from build123d import *

# Parameters (mm, degrees)
BOSS_EXTRUDE1_DEPTH     = 6.35
CUT_EXTRUDE1_DEPTH      = 72.114330131
CUT_EXTRUDE1_DEPTH_BACK = 72.114330131
SKETCH2_R               = 3.175
SCALE1_SCALE            = 4


with BuildPart() as part:
    # Sketch1 → Boss-Extrude1 (new body)
    with BuildSketch(Plane.XY):
        with BuildLine():
            Line((-63.5, 6.985), (63.5, 6.985))
            ThreePointArc((63.5, 6.985), (70.485, 0), (63.5, -6.985))
            Line((63.5, -6.985), (-63.5, -6.985))
            ThreePointArc((-63.5, -6.985), (-70.485, 0), (-63.5, 6.985))
        make_face()
    extrude(amount=BOSS_EXTRUDE1_DEPTH)

    # Sketch2 → Cut-Extrude1 (cut, two sides: drawn at the far end of the back side and taken through both)
    with BuildSketch(Plane.XY.offset(6.35).offset(-CUT_EXTRUDE1_DEPTH_BACK)):
        with Locations((63.5, 0)):
            Circle(SKETCH2_R)
        with Locations((-63.5, 0)):
            Circle(SKETCH2_R)
    extrude(amount=CUT_EXTRUDE1_DEPTH + CUT_EXTRUDE1_DEPTH_BACK, mode=Mode.SUBTRACT)


with BuildPart() as part_1:
    # Scale1: scaled about (0, 0, 3.175)
    add(part.part.scale(SCALE1_SCALE).moved(Location((0, 0, -9.525))))


solid = part_1.part
Check sheet for the modelled part. Datum: model origin and axes. Units: mm. Round coordinates to 2 decimals unless told otherwise and drop trailing zeros. Order: outer loops, then holes, each group sorted by start corner. A loop starts at its lowest first (then second) coordinate and runs counter-clockwise, first axis right, second up. Notation, with made-up numbers: M 76.25,15 L 85.25,15 A19 cw 85.25,23 Z; hole C 77,-26.75 d6. An arc over 180 degrees is marked long. One line per item, written item: value. Start each with the question number.
1. Section check C-C on y = 21. Enter the section's corners in (x, z) (3 decimals).
2. Section check A-A on y = 0. Enter the section's corners in (x, z) (3 decimals).
3. Scan lines: line 1 along X through (y, z) = (-1, 14.25); line 2 along X through (y, z) = (-7.5, -0.25); line 3 along Y through (x, z) = (254, 4.75). Record each from-to range of solid material in increasing order.
4. Gauge pin test, flat ends, axial feed: P1, Ø8, axis at y = -19, z = 4.5, coming from the +X side; P2, Ø1, axis at y = 10, z = -3.5, coming from the -X side; P3, Ø1, axis at y = 7.5, z = 7.5, coming from the -X side. Record the tip position at first contact, or that the pin passes through.
5. Section check B-B on z = -4.5. Enter the section's corners in (x, y), and give its area (3 significant figures).
6. Release check for a two-part mould opening along Y. For faces 1 (the flat face through (4, -27.94, 3)), 2 (the flat face through (4, 0, -9.525)), 3 (the cylindrical face through (266.114, 3.815, 2.997)) record: released by +Y, released by -Y, zero draft, split by the parting line, or undercut.
Results found:
1. outline: M -272.429,-9.525 L 272.429,-9.525 L 272.429,15.875 L -272.429,15.875 Z
2. outline: M -281.94,-9.525 L -266.7,-9.525 L -266.7,15.875 L -281.94,15.875 Z; M -241.3,-9.525 L 241.3,-9.525 L 241.3,15.875 L -241.3,15.875 Z; M 266.7,-9.525 L 281.94,-9.525 L 281.94,15.875 L 266.7,15.875 Z
3. line 1: -281.92 to -266.66, -241.34 to 241.34, 266.66 to 281.92
3. line 2: -280.91 to -264.25, -243.75 to 243.75, 264.25 to 280.91
3. line 3: -27.94 to -12.7, 12.7 to 27.94
4. P1: x = 277.57
4. P2: x = -280.28
4. P3: x = -281.05
5. outline: M -254,-27.94 L 254,-27.94 A27.94 ccw 254,27.94 L -254,27.94 A27.94 ccw Z; hole C -254,0 d25.4; hole C 254,0 d25.4
5. area: 29,800 mm^2
6. face 1: released by -Y
6. face 2: zero draft
6. face 3: undercut
